```python
from build123d import *

# Parameters (mm, degrees)
SKETCH1_W            = 60
SKETCH1_H            = 60
BOSS_EXTRUDE1_DEPTH  = 15
SHELL1_T             = -3
SKETCH2_W            = 6
SKETCH2_H            = 6
BOSS_EXTRUDE2_DEPTH  = 12
LPATTERN1_COUNT      = 2
LPATTERN1_PITCH      = 48
LPATTERN1_COUNT_DIR2 = 2
LPATTERN1_PITCH_DIR2 = 48


with BuildPart() as part:
    # Sketch1 → Boss-Extrude1 (new body)
    with BuildSketch(Plane(origin=(0, 0, 0), x_dir=(1, 0, 0), z_dir=(0, 1, 0))):
        Rectangle(SKETCH1_W, SKETCH1_H)
    extrude(amount=BOSS_EXTRUDE1_DEPTH)

    # Shell1
    shell1_openings = [part.faces().sort_by_distance(p)[0] for p in [
        (0, 15, 0),
    ]]
    offset(amount=SHELL1_T, openings=shell1_openings, kind=Kind.INTERSECTION)

    # Sketch2 → Boss-Extrude2 (add)
    with BuildSketch(Plane(origin=(0, 3, 0), x_dir=(1, 0, 0), z_dir=(0, 1, 0))):
        with Locations((-24, 24)):
            Rectangle(SKETCH2_W, SKETCH2_H)
    boss_extrude2 = extrude(amount=BOSS_EXTRUDE2_DEPTH)

    # LPattern1: Boss-Extrude2 2 × 2
    with Locations(*[(i * LPATTERN1_PITCH, 0, j * LPATTERN1_PITCH_DIR2) for i in range(LPATTERN1_COUNT) for j in range(LPATTERN1_COUNT_DIR2) if (i, j) != (0, 0)]):
        add(boss_extrude2)


solid = part.part
```
Build history of the part. All positions in model axes, mm. A direction names the side the tool comes from. Give positions to 0.01 mm unless a question says otherwise; leave off trailing zeros. Order: outer loops, then holes, each group sorted by start corner. A loop starts at its lowest first (then second) coordinate and runs counter-clockwise, first axis right, second up. Notation, with made-up numbers: M -27.5,83.5 L -5.5,83.5 A31 ccw -5.5,109.5 Z; hole C 67,-39 d8. An arc over 180 degrees is marked long. Return JSON: item names as keys, results as strings.
Q1. Wall check: probe 1 along Z at (x, y) = (-20.5, 6); probe 2 along Z at (x, y) = (26, 10.5). Give the ranges that are in metal, low to high. Write a range as from..to.
Answer list:
{"probe 1": "z = -30..-27, 27..30", "probe 2": "z = -30..-21, 21..30"}
Q2. Band-saw the part on B-B (x = -26). Give the cut face in (y, z).
Answer list:
{"outline": "M 0,-30 L 15,-30 L 15,-21 L 3,-21 L 3,21 L 15,21 L 15,30 L 0,30 Z"}
Q3. Band-saw the part on C-C (z = 24.5). Give the cut face in (x, y), then the cut area to 3 significant figures.
Answer list:
{"outline": "M -30,0 L 30,0 L 30,15 L 21,15 L 21,3 L -21,3 L -21,15 L -30,15 Z", "area": "396 mm^2"}
Q4. Two-plate mould, pull along Z, no slides. Class faces 3 (the face through (0, 7, -30)), 4 (the face through (-30, 7, 0)), 5 (the face through (0, 9, -27)): pulls with the +Z half, pulls with the -Z half, needs draft (parallel to the pull), parting line crosses it, or undercut.
Answer list:
{"face 3": "pulls with the -Z half", "face 4": "needs draft", "face 5": "undercut"}
Q5. 3-axis set-ups, long thin cutter, end or side, ignore diameter. For faces 1 (the face through (0, 7, 30)), 2 (the face through (24, 9, -21)): which of +Z, -Z, +X, -X, +Y, -Y reach the whole face in a straight line?
Answer list:
{"face 1": "+Z, +X, -X, +Y, -Y", "face 2": "+Y"}
Q6. Flat gauge pin, fed straight in: pin 1 (1 mm diameter, centred on x = -3.5, z = -12.5, fed in from -Y). Where does the tip first touch, or does it go through?
Answer list:
{"pin 1": "stops at y = 0"}
Q7. Band-saw the part on A-A (y = 14). Give the cut face in (x, z), then the cut area to 3 significant figures.
Answer list:
{"outline": "M -30,-30 L 30,-30 L 30,30 L -30,30 Z; hole M -27,-21 L -21,-21 L -21,-27 L 21,-27 L 21,-21 L 27,-21 L 27,21 L 21,21 L 21,27 L -21,27 L -21,21 L -27,21 Z", "area": "828 mm^2"}
